Design review of the part built by this model. Coordinates are the model's own, in mm. A direction names the side the tool comes from. Round coordinates to 2 decimals unless told otherwise and drop trailing zeros. Order: outer loops, then holes, each group sorted by start corner. A loop starts at its lowest first (then second) coordinate and runs counter-clockwise, first axis right, second up.
from build123d import *

# Parameters (mm, degrees)
SKETCH_1_W          = 4.8
SKETCH_1_H          = 17
EXTRUDE_1_DEPTH     = 5
SKETCH_2_R          = 3.1
CUT_EXTRUDE_1_DEPTH = 19.358649188
EXTRUDE_2_DEPTH     = 4.8
FILLET_1_R          = 10
SKETCH_4_R          = 1.5
EXTRUDE_3_DEPTH     = 4


with BuildPart() as part:
    # 草图1 → 凸台-拉伸1 (new body)
    with BuildSketch(Plane.XY):
        with Locations((2.4, 8.5)):
            Rectangle(SKETCH_1_W, SKETCH_1_H)
    extrude(amount=EXTRUDE_1_DEPTH)

    # 草图2 → 切除-拉伸1 (cut, through all)
    with BuildSketch(Plane(origin=(4.8, 0, 0), x_dir=(0, 0, -1), z_dir=(1, 0, 0))):
        with Locations((0, 8.5)):
            Circle(SKETCH_2_R)
    extrude(amount=-CUT_EXTRUDE_1_DEPTH, mode=Mode.SUBTRACT)

    # 草图3 → 凸台-拉伸2 (add)
    with BuildSketch(Plane(origin=(4.8, 0, 0), x_dir=(0, 0, -1), z_dir=(1, 0, 0))):
        with BuildLine():
            Line((-5, 11.81662479), (-5, 5.18337521))
            ThreePointArc((-5, 5.18337521), (-6, 8.5), (-5, 11.81662479))
        make_face()
    extrude(amount=-EXTRUDE_2_DEPTH)

    # 圆角1
    # the kernel refuses this fillet: 10 mm, written as the material it takes off along each edge
    with BuildSketch(Plane(origin=(-21.650635095, 0, 0), x_dir=(0, 0, 1), z_dir=(1, 0, 0))) as fillet_1_piece_1:
        with BuildLine():
            CenterArc((10, -8.660254038), FILLET_1_R, 120, 60)
            Line((0, -8.660254038), (0, 0))
            Line((0, 0), (5, 0))
        make_face()
    extrude(amount=48.101270189, mode=Mode.SUBTRACT)
    with BuildSketch(Plane(origin=(26.450635095, 17, 0), x_dir=(0, -1, 0), z_dir=(-1, 0, 0))) as fillet_1_piece_2:
        with BuildLine():
            CenterArc((8.660254038, 10), FILLET_1_R, 210, 60)
            Line((0, 5), (0, 0))
            Line((0, 0), (8.660254038, 0))
        make_face()
    extrude(amount=48.101270189, mode=Mode.SUBTRACT)

    # 草图4 → 凸台-拉伸3 (add)
    with BuildSketch(Plane.XY.offset(5)):
        with Locations(Location((2.4, 13, 0), (0, 0, 232.08440029))):
            Circle(SKETCH_4_R)
        with Locations(Location((2.4, 4, 0), (0, 0, 127.91559971))):
            Circle(SKETCH_4_R)
    extrude(amount=EXTRUDE_3_DEPTH)


solid = part.part
1) Take a section at B-B on x = 1.2. Give the boundary of the cut face in (y, z).
Results:
outline: (0, 5) arc R10 ccw to (5.45, 0.53) arc R3.1 cw to (11.55, 0.53) arc R10 ccw to (17, 5) - (13.9, 5) - (13.9, 9) - (12.1, 9) - (12.1, 5) - (11.82, 5) arc R6 ccw to (5.18, 5) - (4.9, 5) - (4.9, 9) - (3.1, 9) - (3.1, 5) - close
2) To check wall thickness, follow line 1 along Y through (x, z) = (3.4, 8.5); line 2 along X through (y, z) = (4, 6.5); line 3 along Y through (x, z) = (0.8, 1.5). State the ranges of each line that lie inside material, in increasing order.
Results:
line 1: y = 2.88 to 5.12, 11.88 to 14.12
line 2: x = 0.9 to 3.9
line 3: y = 3.39 to 5.79, 11.21 to 13.61
3) Take a section at A-A on z = 2.75. Give the boundary of the cut face in (x, y).
Results:
outline: (0, 1.77) - (4.8, 1.77) - (4.8, 7.07) - (0, 7.07) - close; (0, 9.93) - (4.8, 9.93) - (4.8, 15.23) - (0, 15.23) - close
4) Take a section at D-D on z = 4.5. Give the boundary of the cut face in (x, y).
Results:
outline: (0, 0.31) - (4.8, 0.31) - (4.8, 16.69) - (0, 16.69) - close
5) For faces 1 (the face through (3.3, 2.8, 7)), 2 (the face through (2.4, 8.6, 3.1)), list the 3-axis set-ups (+Z, -Z, +X, -X, +Y, -Y) from which the entire face can be reached by the end or side of a thin tool; tool diameter is ignored.
Results:
face 1: +Z
face 2: -Z, +X, -X
6) Take a section at C-C on y = 13. Give the boundary of the cut face in (x, z).
Results:
outline: (0, 1.15) - (4.8, 1.15) - (4.8, 5) - (3.9, 5) - (3.9, 9) - (0.9, 9) - (0.9, 5) - (0, 5) - close
7) The part is to be moulded in two halves that separate along Y. For faces 3 (the face through (2.43, 14.72, 2.3)), 4 (the face through (2.37, 2.28, 2.3)), 5 (the face through (2.4, 8.5, 6)), say which applies: released by +Y, released by -Y, zero draft, split by the parting line, or undercut.
Results:
face 3: released by +Y
face 4: released by -Y
face 5: undercut
